Source: CAD feature listing. Evaluate the final solid. Frame: model axes, mm. A direction names the side the tool comes from. Coordinates: 2 decimals unless noted, no trailing zeros. Write each loop counter-clockwise with the first axis right and the second up, starting at its lowest first coordinate (ties: lowest second). Pieces come first, ordered by that corner, then holes. Notation, with made-up numbers: (89, 15.25) - (146, 15.25) arc R21 cw to (146, 42.25) - close; hole circle Ø5 at (86, 33). An arc over 180 degrees is marked (long way). One line per question, with ' | ' between items.
from build123d import *

# Parameters (mm, degrees)
BOSS_EXTRUDE1_DEPTH            = 12
BOSS_EXTRUDE1_DEPTH_BACK       = 7
SKETCH1_R                      = 4.915
BOSS_EXTRUDE2_DEPTH            = 12
BOSS_EXTRUDE2_DEPTH_BACK       = 7
SKETCH1_3_W                    = 80
SKETCH1_3_H                    = 5
CUT_EXTRUDE1_REACH             = 103.367
SKETCH2_R                      = 2
CUT_EXTRUDE2_REACH             = 67.146
CUT_EXTRUDE2_DIRECTION_2_REACH = 67.146
FILLET3_R                      = 8.5
FILLET4_R                      = 5.5


with BuildPart() as part:
    # Sketch1 → Boss-Extrude1 (new, two sides: drawn at the far end of the back side and taken through both)
    with BuildSketch(Plane.XY.offset(-BOSS_EXTRUDE1_DEPTH_BACK)):
        Polygon((7.991845682, 47.36466233), (-7.991845682, 47.36466233), (-29.227261436, -45), (29.227261436, -45), align=None)
        with Locations((0, 27.36466233)):
            Circle(SKETCH1_R, mode=Mode.SUBTRACT)
    extrude(amount=BOSS_EXTRUDE1_DEPTH + BOSS_EXTRUDE1_DEPTH_BACK)

    # Sketch1<3> → Boss-Extrude2 (add, two sides: drawn at the far end of the back side and taken through both)
    with BuildSketch(Plane.XY.offset(-BOSS_EXTRUDE2_DEPTH_BACK)):
        with Locations((0, -47.5)):
            Rectangle(SKETCH1_3_W, SKETCH1_3_H)
    extrude(amount=BOSS_EXTRUDE2_DEPTH + BOSS_EXTRUDE2_DEPTH_BACK)

    # Sketch2 → Cut-Extrude1 (cut, up to next)
    with BuildSketch(Plane(origin=(0, -45, 0), x_dir=(1, 0, 0), z_dir=(0, 1, 0)), mode=Mode.PRIVATE) as cut_extrude1_sk1:
        with Locations(Location((-35, 2, 0), (0, 0, 270))):
            Circle(SKETCH2_R)
    cut_extrude1_tool1 = extrude(cut_extrude1_sk1.sketch, amount=-CUT_EXTRUDE1_REACH, mode=Mode.PRIVATE) & part.part
    # Sketch2 → Cut-Extrude1 (cut, up to next)
    with BuildSketch(Plane(origin=(0, -45, 0), x_dir=(1, 0, 0), z_dir=(0, 1, 0)), mode=Mode.PRIVATE) as cut_extrude1_sk2:
        with Locations(Location((-35, -7, 0), (0, 0, 270))):
            Circle(SKETCH2_R)
    cut_extrude1_tool2 = extrude(cut_extrude1_sk2.sketch, amount=-CUT_EXTRUDE1_REACH, mode=Mode.PRIVATE) & part.part
    # Sketch2 → Cut-Extrude1 (cut, up to next)
    with BuildSketch(Plane(origin=(0, -45, 0), x_dir=(1, 0, 0), z_dir=(0, 1, 0)), mode=Mode.PRIVATE) as cut_extrude1_sk3:
        with Locations(Location((35, 2, 0), (0, 0, 270))):
            Circle(SKETCH2_R)
    cut_extrude1_tool3 = extrude(cut_extrude1_sk3.sketch, amount=-CUT_EXTRUDE1_REACH, mode=Mode.PRIVATE) & part.part
    # Sketch2 → Cut-Extrude1 (cut, up to next)
    with BuildSketch(Plane(origin=(0, -45, 0), x_dir=(1, 0, 0), z_dir=(0, 1, 0)), mode=Mode.PRIVATE) as cut_extrude1_sk4:
        with Locations(Location((35, -7, 0), (0, 0, 270))):
            Circle(SKETCH2_R)
    cut_extrude1_tool4 = extrude(cut_extrude1_sk4.sketch, amount=-CUT_EXTRUDE1_REACH, mode=Mode.PRIVATE) & part.part
    add(cut_extrude1_tool1.solids().sort_by_distance((-35, -45, -2))[0], mode=Mode.SUBTRACT)
    add(cut_extrude1_tool2.solids().sort_by_distance((-35, -45, 7))[0], mode=Mode.SUBTRACT)
    add(cut_extrude1_tool3.solids().sort_by_distance((35, -45, -2))[0], mode=Mode.SUBTRACT)
    add(cut_extrude1_tool4.solids().sort_by_distance((35, -45, 7))[0], mode=Mode.SUBTRACT)

    # Sketch3 → Cut-Extrude2 (cut, up to next)
    with BuildSketch(Plane.XY, mode=Mode.PRIVATE) as cut_extrude2_sk1:
        Polygon((-12.48657179, 5.499434813), (12.48657179, 5.499434813), (24.096818248, -45), (-24.096818248, -45), align=None)
    cut_extrude2_tool1 = extrude(cut_extrude2_sk1.sketch, amount=-CUT_EXTRUDE2_REACH, mode=Mode.PRIVATE) & part.part
    add(cut_extrude2_tool1.solids().sort_by_distance((0, -22.421399, 0))[0], mode=Mode.SUBTRACT)

    # Sketch3 → Cut-Extrude2 direction 2 (cut, up to next)
    with BuildSketch(Plane.XY, mode=Mode.PRIVATE) as cut_extrude2_direction_2_sk1:
        Polygon((-12.48657179, 5.499434813), (12.48657179, 5.499434813), (24.096818248, -45), (-24.096818248, -45), align=None)
    cut_extrude2_direction_2_tool1 = extrude(cut_extrude2_direction_2_sk1.sketch, amount=CUT_EXTRUDE2_DIRECTION_2_REACH, mode=Mode.PRIVATE) & part.part
    add(cut_extrude2_direction_2_tool1.solids().sort_by_distance((0, -22.421399, 0))[0], mode=Mode.SUBTRACT)

    # Fillet3
    fillet3_edges = [part.edges().sort_by_distance(p)[0] for p in [
        (-7.991845682, 47.36466233, 2.5),
        (7.991845682, 47.36466233, 2.5),
    ]]
    fillet(fillet3_edges, radius=FILLET3_R)

    # Fillet4
    fillet4_edges = [part.edges().sort_by_distance(p)[0] for p in [
        (-12.48657179, 5.499434813, 2.5),
        (-24.096818248, -45, 2.5),
        (24.096818248, -45, 2.5),
        (12.48657179, 5.499434813, 2.5),
    ]]
    fillet(fillet4_edges, radius=FILLET4_R)


solid = part.part
Item 1: Cut plane A-A on x = 35. Return loops of the section in (y, z).
Check sheet entries:
outline: (-50, -7) - (-45, -7) - (-45, -4) - (-50, -4) - close; (-50, 0) - (-45, 0) - (-45, 5) - (-50, 5) - close; (-50, 9) - (-45, 9) - (-45, 12) - (-50, 12) - close
Item 2: Pin query (flat end, axial travel): pin 1 Ø1 at (y, z) = (21, -4.5) entering from +X; pin 2 Ø8 at (x, y) = (0, 27.36) entering from +Z; pin 3 Ø1.5 at (y, z) = (24, -0.5) entering from -X; pin 4 Ø4 at (y, z) = (16, -2) entering from +X. Return the tip coordinate at first contact, or that it passes through.
Check sheet entries:
pin 1: x = 14.17 | pin 2: through | pin 3: x = -13.54 | pin 4: x = 15.66
Item 3: Access query for faces 4 (the face through (35, -45, 2)), 5 (the face through (17.945, -18.241, 2.633)), 6 (the face through (40, -48, 2)). Directions: +Z, -Z, +X, -X, +Y, -Y. A direction counts if a zero-diameter tool reaches every point of the face in a straight line with its end or side. Return the directions, or none.
Check sheet entries:
face 4: +Z, -Z, +X, +Y | face 5: +Z, -Z | face 6: +Z, -Z, +X, +Y, -Y
Item 4: Cut plane B-B on z = -2. Return loops of the section in (x, y) (3 decimals).
Check sheet entries:
outline: (-40, -50) - (-37, -50) - (-37, -45) - (-40, -45) - close; (-33, -50) - (33, -50) - (33, -45) - (29.227, -45) - (9.508, 40.769) arc R8.5 ccw to (1.224, 47.365) - (-1.224, 47.365) arc R8.5 ccw to (-9.508, 40.769) - (-29.227, -45) - (-33, -45) - close; (37, -50) - (40, -50) - (40, -45) - (37, -45) - close; hole (-22.549, -38.268) arc R5.5 ccw to (-17.189, -45) - (17.189, -45) arc R5.5 ccw to (22.549, -38.268) - (13.468, 1.232) arc R5.5 ccw to (8.108, 5.499) - (-8.108, 5.499) arc R5.5 ccw to (-13.468, 1.232) - close; hole circle Ø9.83 at (0, 27.365)
Item 5: Cut plane D-D on x = 0. Return loops of the section in (y, z).
Check sheet entries:
outline: (-50, -7) - (-45, -7) - (-45, 12) - (-50, 12) - close; (5.5, -7) - (22.45, -7) - (22.45, 12) - (5.5, 12) - close; (32.28, -7) - (47.36, -7) - (47.36, 12) - (32.28, 12) - close
Item 6: Cut plane C-C on y = 30.5. Return loops of the section in (x, z), and give its area (3 significant figures).
Check sheet entries:
outline: (-11.87, -7) - (-3.79, -7) - (-3.79, 12) - (-11.87, 12) - close; (3.79, -7) - (11.87, -7) - (11.87, 12) - (3.79, 12) - close | area: 307 mm²
Item 7: Ray query, line 1 along X through (y, z) = (-48.85, -2); line 2 along Y through (x, z) = (-30, -0.5); line 3 along X through (y, z) = (-33, -3). Return the intervals inside material, ascending. Write a range as [from, to].
Check sheet entries:
line 1: [-40, -37], [-33, 33], [37, 40] | line 2: [-50, -45] | line 3: [-26.47, -21.34], [21.34, 26.47]
Item 8: Mould query, pull axis X, two halves, no side actions, for faces 1 (the face through (-11.574, 4.27, 2.367)), 2 (the face through (0, 47.365, 2)), 3 (the face through (-6.46, 45.56, 2.63)). Classes: pulls with the +X half, pulls with the -X half, needs draft (parallel to the pull), parting line crosses it, or undercut.
Check sheet entries:
face 1: undercut | face 2: needs draft | face 3: pulls with the -X half
